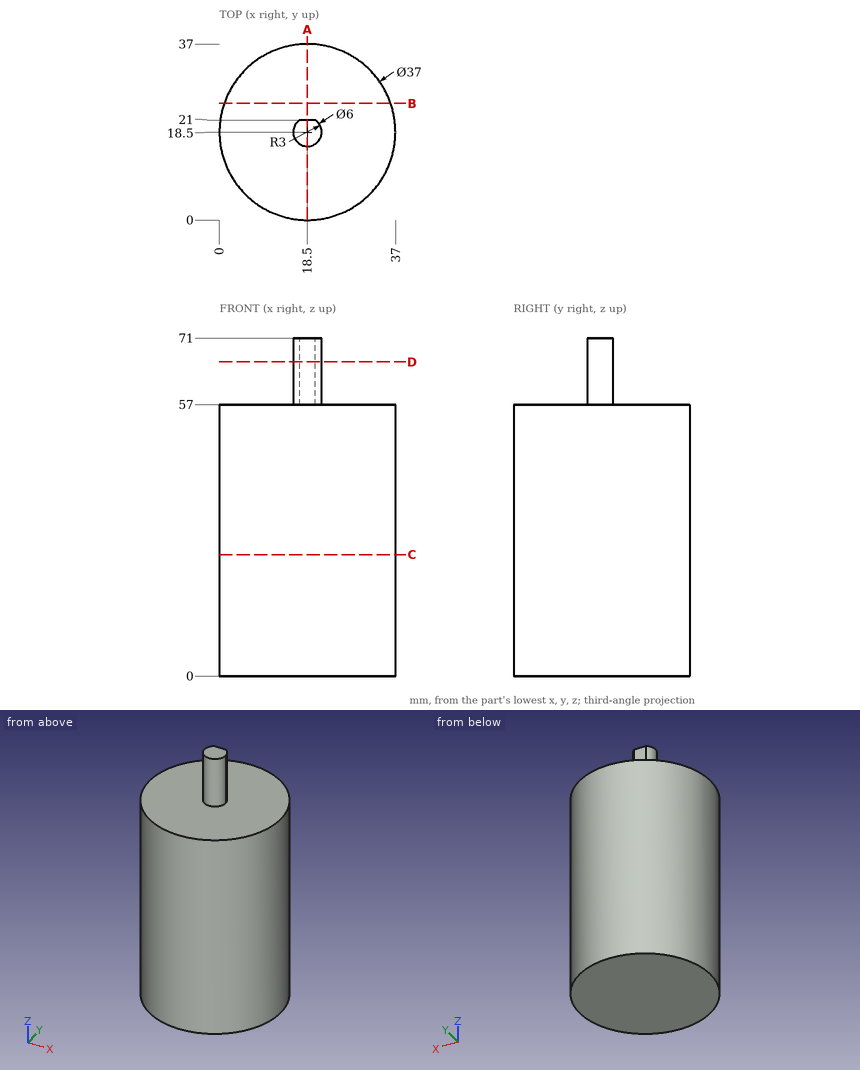
Drawing for the job (mm, zero at the part's lowest x, y, z). Round coordinates to 2 decimals unless told otherwise and drop trailing zeros. Write each loop counter-clockwise with the first axis right and the second up, starting at its lowest first coordinate (ties: lowest second). Pieces come first, ordered by that corner, then holes. Notation, with made-up numbers: (77.5, 83.5) - (131.5, 83.5) arc R21 cw to (131.5, 112.5) - close; hole circle Ø6 at (85, 75.25). An arc over 180 degrees is marked (long way). Return JSON: item names as keys, results as strings. Group by question number.
Item 1: Probe probe 1 along Y at (x, z) = (18, 52.5); probe 2 along Z at (x, y) = (26, 23); probe 3 along X at (y, z) = (14, 46). List the from-to ranges inside material, lowest first.
Item 2: Flat gauge pins, fed straight in: pin 1 Ø12 at (y, z) = (6.5, 16.5) entering from -X; pin 2 Ø5 at (x, z) = (27, 51.5) entering from +Y; pin 3 Ø4 at (x, z) = (12.5, 56) entering from +Y. Where does each tip first touch, or does it go through?
Item 3: Band-saw the part on B-B on y = 24.5. List the corners of the cut face in (x, z), plus the area to 4 significant figures.
Item 4: Band-saw the part on A-A on x = 18.5. List the corners of the cut face in (y, z), plus the area to 3 significant figures.
Item 5: Band-saw the part on D-D on z = 66. List the corners of the cut face in (x, y), plus the area to 3 significant figures.
Item 6: Band-saw the part on C-C on z = 25.5. List the corners of the cut face in (x, y).
Resolved:
{
 "1": {"probe 1": "y = 0.01 to 36.99", "probe 2": "z = 0 to 57", "probe 3": "x = 0.56 to 36.44"},
 "2": {"pin 1": "stops at x = 1", "pin 2": "stops at y = 36", "pin 3": "stops at y = 36.56"},
 "3": {"outline": "(1, 0) - (36, 0) - (36, 57) - (1, 57) - close", "area": "1,995 mm²"},
 "4": {"outline": "(0, 0) - (37, 0) - (37, 57) - (21, 57) - (21, 71) - (15.5, 71) - (15.5, 57) - (0, 57) - close", "area": "2,190 mm²"},
 "5": {"outline": "(16.84, 21) arc R3 ccw (long way) to (20.16, 21) - close", "area": "27.1 mm²"},
 "6": {"outline": "circle Ø37 at (18.5, 18.5)"}
}
